from build123d import *

# Parameters (mm, degrees)
BOSS_EXTRUDE1_DEPTH     = 27
CHAMFER1_SIZE           = 3
SHELL1_T                = -1
CUT_EXTRUDE1_REACH      = 131.009
SKETCH2_W               = 14
SKETCH2_H               = 25
BOSS_EXTRUDE2_DEPTH     = 4
SKETCH7_R               = 1.5
CUT_EXTRUDE2_DEPTH      = 3
MIRROR2_COPY_1_DEPTH    = 4
MIRROR2_COPY_2_SKETCH_R = 1.5
MIRROR2_COPY_2_DEPTH    = 3
CHAMFER2_SIZE           = 2
CHAMFER3_SIZE           = 4


with BuildPart() as part:
    # Sketch1 → Boss-Extrude1 (new body)
    with BuildSketch(Plane.XY):
        with BuildLine():
            Line((54.711561383, -75.098685124), (54.711561383, -31.098685124))
            ThreePointArc((54.711561383, -31.098685124), (51.87049716, -24.239749346), (45.011561383, -21.398685124))
            Line((45.011561383, -21.398685124), (-28.988438617, -21.398685124))
            ThreePointArc((-28.988438617, -21.398685124), (-35.847374395, -24.239749346), (-38.688438617, -31.098685124))
            Line((-38.688438617, -31.098685124), (-38.688438617, -75.098685124))
            ThreePointArc((-38.688438617, -75.098685124), (-35.847374395, -81.957620901), (-28.988438617, -84.798685124))
            Line((-28.988438617, -84.798685124), (45.011561383, -84.798685124))
            ThreePointArc((45.011561383, -84.798685124), (51.87049716, -81.957620901), (54.711561383, -75.098685124))
        make_face()
    extrude(amount=BOSS_EXTRUDE1_DEPTH)

    # Chamfer1
    chamfer1_edges = [part.edges().sort_by_distance(p)[0] for p in [
        (-35.847374395, -24.239749346, 27),
        (-38.688438617, -53.098685124, 27),
        (-35.847374395, -81.957620901, 27),
        (8.011561383, -84.798685124, 27),
        (51.87049716, -81.957620901, 27),
        (54.711561383, -53.098685124, 27),
        (51.87049716, -24.239749346, 27),
        (8.011561383, -21.398685124, 27),
    ]]
    chamfer(chamfer1_edges, length=CHAMFER1_SIZE)

    # Shell1
    shell1_openings = [part.faces().sort_by_distance(p)[0] for p in [
        (8.011561383, -53.098685124, 0),
    ]]
    offset(amount=SHELL1_T, openings=shell1_openings, kind=Kind.INTERSECTION)

    # Sketch2 → Cut-Extrude1 (cut, up to next)
    with BuildSketch(Plane(origin=(54.711561383, 0, 0), x_dir=(0, 0, -1), z_dir=(1, 0, 0)), mode=Mode.PRIVATE) as cut_extrude1_sk1:
        with Locations((-12, -53.098685124)):
            Rectangle(SKETCH2_W, SKETCH2_H)
    cut_extrude1_tool1 = extrude(cut_extrude1_sk1.sketch, amount=-CUT_EXTRUDE1_REACH, mode=Mode.PRIVATE) & part.part
    add(cut_extrude1_tool1.solids().sort_by_distance((54.711561, -53.098685, 12))[0], mode=Mode.SUBTRACT)

    # Sketch3 → Boss-Extrude2 (add)
    with BuildSketch(Plane(origin=(0, 0, 0), x_dir=(-1, 0, 0), z_dir=(0, 0, -1))):
        with BuildLine():
            Line((-54.118192185, -30.956291213), (-48.694716552, -30.956291213))
            Line((-48.694716552, -30.956291213), (-48.694716552, -23.033750656))
            ThreePointArc((-48.694716552, -23.033750656), (-52.633018075, -26.155361191), (-54.118192185, -30.956291213))
        make_face()
    boss_extrude2 = extrude(amount=-BOSS_EXTRUDE2_DEPTH)

    # Sketch7 → Cut-Extrude2 (cut)
    with BuildSketch(Plane(origin=(0, 0, 0), x_dir=(-1, 0, 0), z_dir=(0, 0, -1))):
        with Locations((-50.633416054, -28.397006104)):
            Circle(SKETCH7_R)
    cut_extrude2 = extrude(amount=-CUT_EXTRUDE2_DEPTH, mode=Mode.SUBTRACT)

    # Mirror1: Boss-Extrude2, Cut-Extrude2 across plane
    add(boss_extrude2.mirror(Plane(origin=(0, -53.098685124, 0), x_dir=(0, 0, 1), z_dir=(0, -1, 0))))
    add(cut_extrude2.mirror(Plane(origin=(0, -53.098685124, 0), x_dir=(0, 0, 1), z_dir=(0, -1, 0))), mode=Mode.SUBTRACT)

    # Mirror2: Boss-Extrude2, Cut-Extrude2 across plane
    add(boss_extrude2.mirror(Plane.ZY.offset(-8.011561383)))
    add(cut_extrude2.mirror(Plane.ZY.offset(-8.011561383)), mode=Mode.SUBTRACT)

    # Mirror2 copy 1 sketch → Mirror2 copy 1 (add)
    with BuildSketch(Plane(origin=(16.023122766, -106.197370247, 0), x_dir=(1, 0, 0), z_dir=(0, 0, -1))):
        with BuildLine():
            Line((-54.118192185, -30.956291213), (-48.694716552, -30.956291213))
            Line((-48.694716552, -30.956291213), (-48.694716552, -23.033750656))
            ThreePointArc((-48.694716552, -23.033750656), (-52.633018075, -26.155361191), (-54.118192185, -30.956291213))
        make_face()
    extrude(amount=-MIRROR2_COPY_1_DEPTH)

    # Mirror2 copy 2 sketch → Mirror2 copy 2 (cut)
    with BuildSketch(Plane(origin=(16.023122766, -106.197370247, 0), x_dir=(1, 0, 0), z_dir=(0, 0, -1))):
        with Locations((-50.633416054, -28.397006104)):
            Circle(MIRROR2_COPY_2_SKETCH_R)
    extrude(amount=-MIRROR2_COPY_2_DEPTH, mode=Mode.SUBTRACT)

    # Chamfer2
    chamfer2_edges = [part.edges().sort_by_distance(p)[0] for p in [
        (48.694716552, -30.956291213, 2),
        (48.694716552, -75.241079034, 2),
        (-32.671593786, -75.241079034, 2),
        (-32.671593786, -30.956291213, 2),
    ]]
    chamfer(chamfer2_edges, length=CHAMFER2_SIZE)

    # Chamfer3
    # the kernel refuses this chamfer: 4 mm, written as the material it adds along each edge
    with BuildSketch(Plane(origin=(-28.988438617, -31.098685124, 4), x_dir=(-0.39359677864958253, -0.9192831858772744, 0), z_dir=(0.9192831858772744, -0.39359677864958253, 0))) as chamfer3_piece_1_section:
        Polygon((8.7, -CHAMFER3_SIZE), (8.7 - CHAMFER3_SIZE, 0), (8.7, 0), align=None)
    chamfer3_piece_1 = revolve(axis=Axis((-28.988438617, -31.098685124, 4), (0, 0, -1)), revolution_arc=199.53449135, mode=Mode.PRIVATE)
    chamfer3_piece_1 = split(chamfer3_piece_1, bisect_by=Plane(origin=(-32.671593786, -27.350508509, 5.442527719), z_dir=(-1, 0, 0)), keep=Keep.TOP, mode=Mode.PRIVATE)
    chamfer3_piece_1 = split(chamfer3_piece_1, bisect_by=Plane(origin=(-35.212045354, -30.956291213, 5.442527719), z_dir=(0, 1, 0)), keep=Keep.TOP, mode=Mode.PRIVATE)
    chamfer3_piece_1 = split(chamfer3_piece_1, bisect_by=Plane(origin=(-33.138928218, -29.423625644, 5.442527719), z_dir=(-0.7071067811865476, 0.7071067811865476, 0)), keep=Keep.TOP, mode=Mode.PRIVATE)
    add(chamfer3_piece_1)
    with BuildSketch(Plane(origin=(-28.988438617, -75.098685124, 4), x_dir=(0.6783261272249539, -0.7347609578114475, 0), z_dir=(0.7347609578114475, 0.6783261272249539, 0))) as chamfer3_piece_2_section:
        Polygon((8.7, -CHAMFER3_SIZE), (8.7 - CHAMFER3_SIZE, 0), (8.7, 0), align=None)
    chamfer3_piece_2 = revolve(axis=Axis((-28.988438617, -75.098685124, 4), (0, 0, -1)), revolution_arc=199.53449135, mode=Mode.PRIVATE)
    chamfer3_piece_2 = split(chamfer3_piece_2, bisect_by=Plane(origin=(-35.212045354, -75.241079034, 5.44252772), z_dir=(0, -1, 0)), keep=Keep.TOP, mode=Mode.PRIVATE)
    chamfer3_piece_2 = split(chamfer3_piece_2, bisect_by=Plane(origin=(-32.671593786, -78.846861739, 5.44252772), z_dir=(-1, 0, 0)), keep=Keep.TOP, mode=Mode.PRIVATE)
    chamfer3_piece_2 = split(chamfer3_piece_2, bisect_by=Plane(origin=(-33.138928218, -76.773744603, 5.44252772), z_dir=(-0.7071067811865476, -0.7071067811865476, 0)), keep=Keep.TOP, mode=Mode.PRIVATE)
    add(chamfer3_piece_2)
    with BuildSketch(Plane(origin=(45.011561383, -75.098685124, 4), x_dir=(0.39359677864958265, 0.9192831858772744, 0), z_dir=(-0.9192831858772744, 0.39359677864958265, 0))) as chamfer3_piece_3_section:
        Polygon((8.7, -CHAMFER3_SIZE), (8.7 - CHAMFER3_SIZE, 0), (8.7, 0), align=None)
    chamfer3_piece_3 = revolve(axis=Axis((45.011561383, -75.098685124, 4), (0, 0, -1)), revolution_arc=199.53449135, mode=Mode.PRIVATE)
    chamfer3_piece_3 = split(chamfer3_piece_3, bisect_by=Plane(origin=(48.694716552, -78.846861739, 5.44252772), z_dir=(1, 0, 0)), keep=Keep.TOP, mode=Mode.PRIVATE)
    chamfer3_piece_3 = split(chamfer3_piece_3, bisect_by=Plane(origin=(51.23516812, -75.241079034, 5.44252772), z_dir=(0, -1, 0)), keep=Keep.TOP, mode=Mode.PRIVATE)
    chamfer3_piece_3 = split(chamfer3_piece_3, bisect_by=Plane(origin=(49.162050984, -76.773744603, 5.44252772), z_dir=(0.7071067811865476, -0.7071067811865476, 0)), keep=Keep.TOP, mode=Mode.PRIVATE)
    add(chamfer3_piece_3)
    with BuildSketch(Plane(origin=(45.011561383, -31.098685124, 4), x_dir=(-0.6783261272249526, 0.7347609578114488, 0), z_dir=(-0.7347609578114488, -0.6783261272249526, 0))) as chamfer3_piece_4_section:
        Polygon((8.7, -CHAMFER3_SIZE), (8.7 - CHAMFER3_SIZE, 0), (8.7, 0), align=None)
    chamfer3_piece_4 = revolve(axis=Axis((45.011561383, -31.098685124, 4), (0, 0, -1)), revolution_arc=199.53449135, mode=Mode.PRIVATE)
    chamfer3_piece_4 = split(chamfer3_piece_4, bisect_by=Plane(origin=(51.23516812, -30.956291213, 5.44252772), z_dir=(0, 1, 0)), keep=Keep.TOP, mode=Mode.PRIVATE)
    chamfer3_piece_4 = split(chamfer3_piece_4, bisect_by=Plane(origin=(49.162050984, -29.423625644, 5.44252772), z_dir=(0.7071067811865476, 0.7071067811865476, 0)), keep=Keep.TOP, mode=Mode.PRIVATE)
    chamfer3_piece_4 = split(chamfer3_piece_4, bisect_by=Plane(origin=(48.694716552, -27.350508508, 5.44252772), z_dir=(1, 0, 0)), keep=Keep.TOP, mode=Mode.PRIVATE)
    add(chamfer3_piece_4)


solid = part.part
The listing builds one solid part. Answer for the finished solid, in the listing's coordinates (mm). A direction names the side the tool comes from. Coordinates: 2 decimals unless noted, no trailing zeros. Order: outer loops, then holes, each group sorted by start corner. A loop starts at its lowest first (then second) coordinate and runs counter-clockwise, first axis right, second up.
Q1. For a pull along X with two mould halves and no side action, classify faces 1 (the face through (51.739, -27.383, 1.479)), 2 (the face through (51.795, -82.033, 11.832)), 3 (the face through (9, -21.399, 12)) as pulls with the +X half, pulls with the -X half, needs draft (parallel to the pull), parting line crosses it, or undercut.
Q2. Which of the six approach directions +Z, -Z, +X, -X, +Y, -Y give full straight-line access (tool end or side, diameter ignored) to faces 4 (the face through (-34.03, -25.95, 25.08)), 5 (the face through (49, -29, 0)), 6 (the face through (51.739, -78.814, 1.479))?
Q3. A cutting plane is placed at C-C, the plane x = 38.5. Write down the section's boundary in (y, z), and give its area (3 significant figures).
Q4. Given P1, Ø3.5, axis at x = -34.5, y = -28.5, coming from the -Z side; P2, Ø3, axis at y = -81.5, z = 4.5, coming from the -X side; P3, Ø8, axis at x = -23, y = -77, coming from the -Z side; P4, Ø4.5, axis at y = -26.5, z = 3.5, coming from the +X side, each flat-ended and moving along its own axis, determine where each tip first touches the part or whether it passes through.
Q5. A cutting plane is placed at D-D, the plane z = 10. Write down the section's boundary in (x, y), and give its area (3 significant figures).
Q6. Consider line 1 (X direction, y = -51, z = 23.5); line 2 (Y direction, x = -26.5, z = 3.5); line 3 (Z direction, x = 39, y = -39). Determine where each line is inside the solid, lowest interval first.
Q7. A cutting plane is placed at A-A, the plane y = -52.5. Write down the section's boundary in (x, z).
Q8. A cutting plane is placed at B-B, the plane z = 20.5. Write down the section's boundary in (x, y).
Answers follow:
1. face 1: undercut
1. face 2: pulls with the +X half
1. face 3: needs draft
2. face 4: none
2. face 5: -Z, +X, -X, +Y, -Y
2. face 6: -Z
3. outline: (-84.8, 0) - (-83.8, 0) - (-83.8, 23.59) - (-81.38, 26) - (-24.81, 26) - (-22.4, 23.59) - (-22.4, 0) - (-21.4, 0) - (-21.4, 24) - (-24.4, 27) - (-81.8, 27) - (-84.8, 24) - close
3. area: 112 mm2
4. P1: stops at z = 0
4. P2: stops at x = -37.36
4. P3: stops at z = 26
4. P4: stops at x = 54.42
5. outline: (-38.69, -75.1) arc R9.7 ccw to (-28.99, -84.8) - (45.01, -84.8) arc R9.7 ccw to (54.71, -75.1) - (54.71, -65.6) - (53.71, -65.6) - (53.71, -75.1) arc R8.7 cw to (45.01, -83.8) - (-28.99, -83.8) arc R8.7 cw to (-37.69, -75.1) - (-37.69, -31.1) arc R8.7 cw to (-28.99, -22.4) - (45.01, -22.4) arc R8.7 cw to (53.71, -31.1) - (53.71, -40.6) - (54.71, -40.6) - (54.71, -31.1) arc R9.7 ccw to (45.01, -21.4) - (-28.99, -21.4) arc R9.7 ccw to (-38.69, -31.1) - close
5. area: 269 mm2
6. line 1: x = -38.69 to -37.69, 53.71 to 54.71
6. line 2: y = -84.8 to -83.8, -22.4 to -21.4
6. line 3: z = 26 to 27
7. outline: (-38.69, 0) - (-37.69, 0) - (-37.69, 23.59) - (-35.27, 26) - (51.3, 26) - (53.71, 23.59) - (53.71, 19) - (54.71, 19) - (54.71, 24) - (51.71, 27) - (-35.69, 27) - (-38.69, 24) - close; (53.71, 0) - (54.71, 0) - (54.71, 5) - (53.71, 5) - close
8. outline: (-38.69, -75.1) arc R9.7 ccw to (-28.99, -84.8) - (45.01, -84.8) arc R9.7 ccw to (54.71, -75.1) - (54.71, -31.1) arc R9.7 ccw to (45.01, -21.4) - (-28.99, -21.4) arc R9.7 ccw to (-38.69, -31.1) - close; hole (-37.69, -75.1) arc R8.7 ccw to (-28.99, -83.8) - (45.01, -83.8) arc R8.7 ccw to (53.71, -75.1) - (53.71, -31.1) arc R8.7 ccw to (45.01, -22.4) - (-28.99, -22.4) arc R8.7 ccw to (-37.69, -31.1) - close
